from build123d import *

# Parameters (mm, degrees)
SKETCH2_W                 = 25.4
SKETCH2_H                 = 3
BOSS_EXTRUDE1_DEPTH       = 70
SKETCH4_R                 = 30
BOSS_EXTRUDE2_DEPTH       = 10
SKETCH5_R                 = 30
SKETCH5_R_2               = 20
BOSS_EXTRUDE3_DEPTH       = 70
SKETCH8_R                 = 24.75
SKETCH8_R_2               = 20
BOSS_EXTRUDE4_DEPTH       = 20
SKETCH9_R                 = 1.5
CUT_EXTRUDE4_DEPTH        = 29.5
CUT_EXTRUDE4_DEPTH_BACK   = 32.5
F_4_40_TAPPED_HOLE1_D     = 2.2606
F_4_40_TAPPED_HOLE1_DEPTH = 7.6
F_4_40_TAPPED_HOLE1_TIP   = 0.679152758
SKETCH3_R                 = 3
CUT_EXTRUDE5_DEPTH        = 10
SKETCH12_R                = 27
SKETCH12_R_2              = 20
CUT_EXTRUDE6_DEPTH        = 60


with BuildPart() as part:
    # Sketch2 → Boss-Extrude1 (new body)
    with BuildSketch(Plane(origin=(0, 0, 0), x_dir=(1, 0, 0), z_dir=(0, 1, 0))):
        with Locations((12.7, 1.5)):
            Rectangle(SKETCH2_W, SKETCH2_H)
    extrude(amount=BOSS_EXTRUDE1_DEPTH)

    # Sketch4 → Boss-Extrude2 (add)
    with BuildSketch(Plane(origin=(0, 70, 0), x_dir=(1, 0, 0), z_dir=(0, 1, 0))):
        with Locations((12.7, 1.5)):
            Circle(SKETCH4_R)
    extrude(amount=BOSS_EXTRUDE2_DEPTH)

    # Sketch5 → Boss-Extrude3 (add)
    with BuildSketch(Plane(origin=(0, 80, 0), x_dir=(1, 0, 0), z_dir=(0, 1, 0))):
        with Locations((12.7, 1.5)):
            Circle(SKETCH5_R)
        with Locations((12.7, 1.5)):
            Circle(SKETCH5_R_2, mode=Mode.SUBTRACT)
    extrude(amount=BOSS_EXTRUDE3_DEPTH)

    # Sketch8 → Boss-Extrude4 (add)
    with BuildSketch(Plane(origin=(0, 150, 0), x_dir=(1, 0, 0), z_dir=(0, 1, 0))):
        with Locations((12.7, 1.5)):
            Circle(SKETCH8_R)
        with Locations((12.7, 1.5)):
            Circle(SKETCH8_R_2, mode=Mode.SUBTRACT)
    extrude(amount=BOSS_EXTRUDE4_DEPTH)

    # Sketch9 → Cut-Extrude4 (cut, two sides)
    with BuildSketch(Plane.XY) as cut_extrude4_sk:
        with Locations((12.7, 160)):
            Circle(SKETCH9_R)
    extrude(amount=CUT_EXTRUDE4_DEPTH, mode=Mode.SUBTRACT)
    extrude(cut_extrude4_sk.sketch, amount=-CUT_EXTRUDE4_DEPTH_BACK, mode=Mode.SUBTRACT)

    # #4-40 Tapped Hole1
    with Locations(Plane.XY):
        with Locations((12.7, 22.2), (20.927241336, 17.45), (20.927241336, 7.95), (12.7, 3.2), (4.472758664, 7.95), (4.472758664, 17.45)):
            Hole(F_4_40_TAPPED_HOLE1_D / 2, depth=F_4_40_TAPPED_HOLE1_DEPTH)
            with Locations((0, 0, -(F_4_40_TAPPED_HOLE1_DEPTH + F_4_40_TAPPED_HOLE1_TIP / 2))):  # 118° drill point
                Cone(0, F_4_40_TAPPED_HOLE1_D / 2, F_4_40_TAPPED_HOLE1_TIP, mode=Mode.SUBTRACT)

    # Sketch3 → Cut-Extrude5 (cut)
    with BuildSketch(Plane.XY):
        with Locations((12.7, 12.7)):
            Circle(SKETCH3_R)
    extrude(amount=-CUT_EXTRUDE5_DEPTH, mode=Mode.SUBTRACT)

    # Sketch12 → Cut-Extrude6 (cut)
    with BuildSketch(Plane(origin=(0, 80, 0), x_dir=(1, 0, 0), z_dir=(0, 1, 0))):
        with Locations((12.7, 1.5)):
            Circle(SKETCH12_R)
        with Locations((12.7, 1.5)):
            Circle(SKETCH12_R_2, mode=Mode.SUBTRACT)
    extrude(amount=CUT_EXTRUDE6_DEPTH, mode=Mode.SUBTRACT)


solid = part.part
Model file for the job. Use its own axes, mm. A direction names the side the tool comes from. Round coordinates to 2 decimals unless told otherwise and drop trailing zeros. Loops run counter-clockwise (first coordinate to the right, second up) from the corner with the lowest first, then second, coordinate; pieces in that order, holes last. Notation, with made-up numbers: (46.25, 35.25) - (52.25, 35.25) arc R18 cw to (52.25, 62.25) - close; hole circle Ø1 at (74.5, -15). An arc over 180 degrees is marked (long way). Write each question's results on one line, items separated by ' | '.
(1) Saw through at C-C, the plane y = 93.5. List the corners of the cut face in (x, z), then the cut area to 3 significant figures.
Answer below:
outline: circle Ø60 at (12.7, -1.5); hole circle Ø54 at (12.7, -1.5) | area: 537 mm^2
(2) Saw through at D-D, the plane z = 12.5. List the corners of the cut face in (x, y).
Answer below:
outline: (-13.83, 70) - (39.23, 70) - (39.23, 150) - (33.11, 150) - (33.11, 170) - (26.98, 170) - (26.98, 140) - (35.79, 140) - (35.79, 80) - (-10.39, 80) - (-10.39, 140) - (-1.58, 140) - (-1.58, 170) - (-7.71, 170) - (-7.71, 150) - (-13.83, 150) - close
(3) Mould opens along Z. For faces 1 (the cylindrical face through (10.1, 154.79, -21.33)), 2 (the cylindrical face through (9.48, 159.86, -26.04)), 3 (the flat face through (0, 35, -1)) say: released by +Z, released by -Z, zero draft, split by the parting line, or undercut.
Answer below:
face 1: undercut | face 2: split by the parting line | face 3: zero draft
(4) Wall check: L1, parallel to Y at x = 12.7, z = 21.95; L2, parallel to Y at x = 2.5, z = -25; L3, parallel to Y at x = 12, z = -1. Give the ranges that are in metal, low to high.
Answer below:
L1: y = 70 to 80, 140 to 158.5, 161.5 to 170 | L2: y = 70 to 80, 140 to 150 | L3: y = 0 to 2.31, 4.09 to 9.78, 15.62 to 21.31, 23.09 to 80
(5) 3-axis set-ups, long thin cutter, end or side, ignore diameter. For faces 4 (the flat face through (25.4, 35, -1)), 5 (the flat face through (17, 150, -26.1)), 6 (the flat face through (13, 35, 0)), 7 (the cylindrical face through (25.159, 109.58, 22.454)), 8 (the flat face through (13, 35, -3)): which of +Z, -Z, +X, -X, +Y, -Y reach the whole face in a straight line?
Answer below:
face 4: +Z, -Z, +X, -Y | face 5: +Y | face 6: +Z, +X, -X, -Y | face 7: none | face 8: -Z, +X, -X, -Y
(6) Saw through at B-B, the plane z = -15. List the corners of the cut face in (x, y), then the cut area to 3 significant figures.
Answer below:
outline: (-14.09, 70) - (39.49, 70) - (39.49, 150) - (33.44, 150) - (33.44, 170) - (27.46, 170) - (27.46, 140) - (36.08, 140) - (36.08, 80) - (-10.68, 80) - (-10.68, 140) - (-2.06, 140) - (-2.06, 170) - (-8.04, 170) - (-8.04, 150) - (-14.09, 150) - close | area: 1,420 mm^2
(7) Saw through at A-A, the plane y = 12.7. List the corners of the cut face in (x, z).
Answer below:
outline: (0, -3) - (9.7, -3) - (9.7, 0) - (0, 0) - close; (15.7, -3) - (25.4, -3) - (25.4, 0) - (15.7, 0) - close
(8) Pin check, flat tips, straight feed: pin 1 (3.5 mm diameter, centred on x = 20.93, y = 7.95, fed in from -Z); pin 2 (2.5 mm diameter, centred on x = 12.7, y = 160, fed in from +Z); pin 3 (3 mm diameter, centred on x = 3, z = 10, fed in from -Y); pin 4 (1 mm diameter, centred on x = 23, y = 107.5, fed in from +Z). Stop position of each tip, or through.
Answer below:
pin 1: stops at z = -3 | pin 2: passes through | pin 3: stops at y = 70 | pin 4: stops at z = 26.85
